Drawing for the job (mm, zero at the part's lowest x, y, z). A direction names the side the tool comes from. Coordinates: 2 decimals unless noted, no trailing zeros. Loops run counter-clockwise (first coordinate to the right, second up) from the corner with the lowest first, then second, coordinate; pieces in that order, holes last. Notation, with made-up numbers: (-37, -22.5) - (11, -22.5) arc R33 cw to (11, 15.5) - close; hole circle Ø8 at (-12.5, -40). An arc over 180 degrees is marked (long way). Put each result on its own line as item: value.
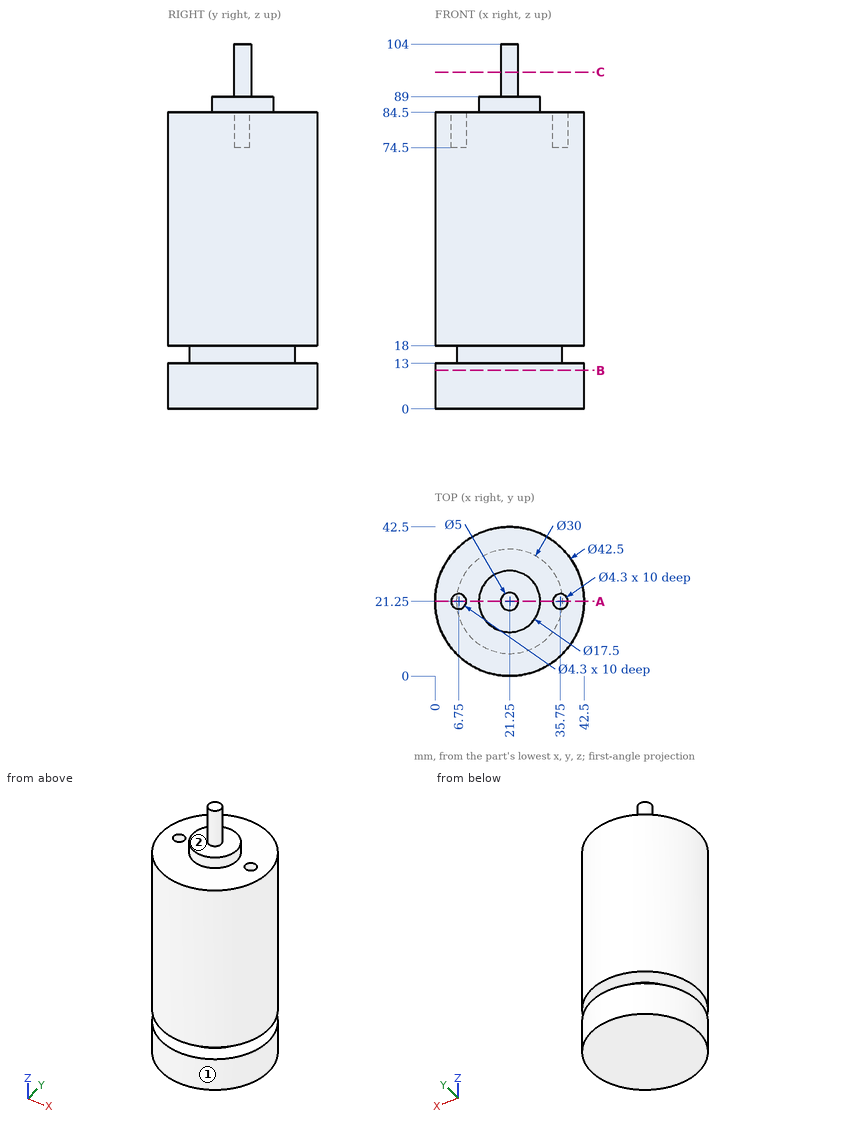
Q1. Slice it at C-C, the plane z = 96. Give the cut face in (x, y), then the cut area to 3 significant figures.
Determined:
outline: circle Ø5 at (21.25, 21.25)
area: 19.6 mm2
Q2. Pin check, flat tips, straight feed: pin 1 Ø4 at (y, z) = (13, 28.5) entering from -X; pin 2 Ø5 at (y, z) = (30, 54) entering from +X; pin 3 Ø4 at (x, z) = (18, 78) entering from -Y. Stop position of each tip, or through.
Determined:
pin 1: x = 0.94
pin 2: x = 41.56
pin 3: y = 0.04
Q3. Wall check: L1, parallel to Z at x = 10, y = 5.5; L2, parallel to Z at x = 30, y = 12.5; L3, parallel to Y at x = 6.75, z = 81.5. Give the ranges that are in metal, low to high. Write a range as from..to.
Determined:
L1: 0..13, 18..84.5
L2: 0..84.5
L3: 5.72..19.1, 23.4..36.78
Q4. Slice it at A-A, the plane y = 21.25. Give the cut face in (x, z).
Determined:
outline: (0, 0) - (42.5, 0) - (42.5, 13) - (36.25, 13) - (36.25, 18) - (42.5, 18) - (42.5, 84.5) - (37.9, 84.5) - (37.9, 74.5) - (33.6, 74.5) - (33.6, 84.5) - (30, 84.5) - (30, 89) - (23.75, 89) - (23.75, 104) - (18.75, 104) - (18.75, 89) - (12.5, 89) - (12.5, 84.5) - (8.9, 84.5) - (8.9, 74.5) - (4.6, 74.5) - (4.6, 84.5) - (0, 84.5) - (0, 18) - (6.25, 18) - (6.25, 13) - (0, 13) - close
Q5. Tool access for the marked faces 1 and 2: list every direction of +Z, -Z, +X, -X, +Y, -Y with a clear straight run to the whole face (end or side of a thin tool).
Determined:
face 1: +Z, -Z
face 2: +Z
Q6. Slice it at B-B, the plane z = 11. Give the cut face in (x, y), then the cut area to 3 significant figures.
Determined:
outline: circle Ø42.5 at (21.25, 21.25)
area: 1,420 mm2
